```python
from build123d import *

# Parameters (mm, degrees)
SKETCH_1_R      = 22.5
EXTRUDE_1_DEPTH = 30
EXTRUDE_2_DEPTH = 10
SKETCH_4_R      = 22.5
EXTRUDE_3_DEPTH = 30


with BuildPart() as part:
    # 草图1 → 凸台-拉伸1 (new body)
    with BuildSketch(Plane.XY):
        Circle(SKETCH_1_R)
    extrude(amount=EXTRUDE_1_DEPTH)

    # 草图3 → 凸台-拉伸2 (add)
    with BuildSketch(Plane.XY.offset(30)):
        with BuildLine():
            Line((-10.048538424, 20.13148965), (-9.44725249, 18.926858585))
            ThreePointArc((-9.44725249, 18.926858585), (0, 21.153641661), (9.44725249, 18.926858585))
            Line((9.44725249, 18.926858585), (10.048538424, 20.13148965))
            ThreePointArc((10.048538424, 20.13148965), (0, 22.5), (-10.048538424, 20.13148965))
        make_face()
        with BuildLine():
            Line((-10.048538424, -20.13148965), (-9.44725249, -18.926858585))
            ThreePointArc((-9.44725249, -18.926858585), (0, -21.153641661), (9.44725249, -18.926858585))
            Line((9.44725249, -18.926858585), (10.048538424, -20.13148965))
            ThreePointArc((10.048538424, -20.13148965), (0, -22.5), (-10.048538424, -20.13148965))
        make_face()
    extrude(amount=EXTRUDE_2_DEPTH)

    # 草图4 → 凸台-拉伸3 (add)
    with BuildSketch(Plane.XY.offset(40)):
        Circle(SKETCH_4_R)
    extrude(amount=EXTRUDE_3_DEPTH)


solid = part.part
```
Here's how the part is built. I have some questions about the finished solid (model axes, mm). A direction names the side the tool comes from. Coordinates: 2 decimals unless noted, no trailing zeros. Loops run counter-clockwise (first coordinate to the right, second up) from the corner with the lowest first, then second, coordinate; pieces in that order, holes last. Notation, with made-up numbers: (24, 42.25) - (40, 42.25) arc R28 cw to (40, 78.25) - close; hole circle Ø11 at (45.25, 47.25). An arc over 180 degrees is marked (long way). Answer as CSV lines item,"result".
Q1. If we section it at B-B, the plane y = 0: Write out the boundary of the cut face in (x, z).
Response:
outline,"(-22.5, 0) - (22.5, 0) - (22.5, 30) - (-22.5, 30) - close; (-22.5, 40) - (22.5, 40) - (22.5, 70) - (-22.5, 70) - close"
Q2. If we section it at C-C, the plane x = -19: Write out the boundary of the cut face in (y, z).
Response:
outline,"(-12.05, 0) - (12.05, 0) - (12.05, 30) - (-12.05, 30) - close; (-12.05, 40) - (12.05, 40) - (12.05, 70) - (-12.05, 70) - close"
Q3. For pin 1 (10 mm diameter, centred on x = 11.5, z = 60, fed in from -Y); pin 2 (5 mm diameter, centred on x = 12, z = 51.5, fed in from +Y); pin 3 (21 mm diameter, centred on x = -6.5, y = 9, fed in from -Z); pin 4 (10 mm diameter, centred on x = 9, z = 18, fed in from +Y), each with a flat end and sliding along its axis, tell me the tip position at first contact or that it passes through.
Response:
pin 1,"y = -21.54"
pin 2,"y = 20.4"
pin 3,"z = 0"
pin 4,"y = 22.14"
Q4. If we section it at A-A, the plane x = 0: Write out the boundary of the cut face in (y, z).
Response:
outline,"(-22.5, 0) - (22.5, 0) - (22.5, 70) - (-22.5, 70) - close; hole (-21.15, 30) - (21.15, 30) - (21.15, 40) - (-21.15, 40) - close"
Q5. If I drill on L1, parallel to Z at x = -6.5, y = -14.5; L2, parallel to X at y = -0.5, z = 15; L3, parallel to Y at x = -5.5, z = 49, over which ranges is the centre line in solid material (lowest first)? Write a range as [from, to].
Response:
L1,"[0, 30], [40, 70]"
L2,"[-22.49, 22.49]"
L3,"[-21.82, 21.82]"
Q6. If we section it at D-D, the plane z = 11: Write out the boundary of the cut face in (x, y), and give its area (3 significant figures).
Response:
outline,"circle Ø45 at (0, 0)"
area,"1,590 mm2"
Q7. For faces 1 (the face through (-0.137, -21.153, 34.93)), 2 (the face through (0, 0, 70)), which set-ups out of +Z, -Z, +X, -X, +Y, -Y let a thin tool reach every point of the face, with its end or its side?
Response:
face 1,"none"
face 2,"+Z, +X, -X, +Y, -Y"
Q8. We'd pull the mould along X, two halves only. Please class faces 3 (the face through (-0.137, 21.153, 34.93)), 4 (the face through (0, 0, 0)): pulls with the +X half, pulls with the -X half, needs draft (parallel to the pull), parting line crosses it, or undercut.
Response:
face 3,"undercut"
face 4,"needs draft"
